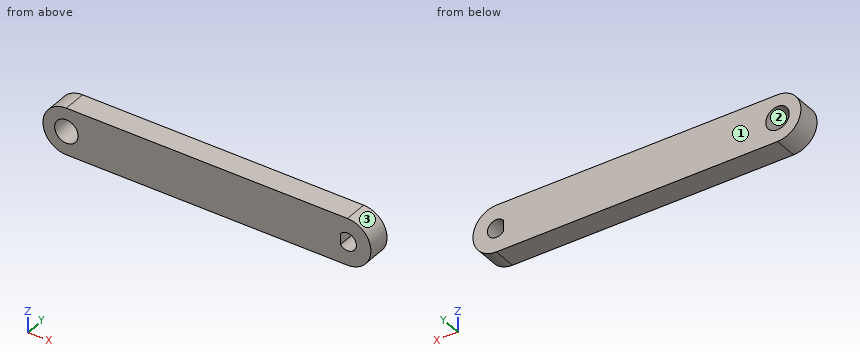
```python
from build123d import *

# Parameters (mm, degrees)
BOSS_EXTRUDE1_DEPTH = 6.35
CUT_EXTRUDE1_DEPTH  = 84.037024874
SKETCH4_R           = 3.175
CUT_EXTRUDE3_DEPTH  = 84.037024874


with BuildPart() as part:
    # Sketch1 → Boss-Extrude1 (new body)
    with BuildSketch(Plane(origin=(0, 0, 0), x_dir=(1, 0, 0), z_dir=(0, 1, 0))):
        with BuildLine():
            Line((0, -6.35), (-76.2, -6.35))
            ThreePointArc((-76.2, -6.35), (-82.55, 0), (-76.2, 6.35))
            Line((-76.2, 6.35), (0, 6.35))
            ThreePointArc((0, 6.35), (6.35, 0), (0, -6.35))
        make_face()
    extrude(amount=BOSS_EXTRUDE1_DEPTH)

    # Sketch2 → Cut-Extrude1 (cut, through all)
    with BuildSketch(Plane(origin=(0, 6.35, 0), x_dir=(1, 0, 0), z_dir=(0, 1, 0))):
        with BuildLine():
            Line((-1.905, -1.481061781), (-1.905, 1.481061781))
            ThreePointArc((-1.905, 1.481061781), (2.413, 0), (-1.905, -1.481061781))
        make_face()
    extrude(amount=-CUT_EXTRUDE1_DEPTH, mode=Mode.SUBTRACT)

    # Sketch4 → Cut-Extrude3 (cut, through all)
    with BuildSketch(Plane(origin=(0, 6.35, 0), x_dir=(1, 0, 0), z_dir=(0, 1, 0))):
        with Locations(Location((-76.2, 0, 0), (0, 0, 270))):
            Circle(SKETCH4_R)
    extrude(amount=-CUT_EXTRUDE3_DEPTH, mode=Mode.SUBTRACT)


solid = part.part
```
Build history of the part. All positions in model axes, mm. Face numbers are marked on the shaded views. Give positions to 0.01 mm unless a question says otherwise; leave off trailing zeros. Order: outer loops, then holes, each group sorted by start corner. A loop starts at its lowest first (then second) coordinate and runs counter-clockwise, first axis right, second up. Notation, with made-up numbers: M 26,-33 L 84,-33 A30 cw 84,-4 Z; hole C -38.5,36 d6. An arc over 180 degrees is marked long. Write item = value, one per line. Start each with the question number.
(1) Slice it at B-B on y = 1.5. Write the cut outline in (x, z) (3 decimals).
(2) Pin check, flat tips, straight feed: pin 1 Ø5 at (x, z) = (-76.2, 0) entering from +Y; pin 2 Ø1 at (y, z) = (3, 4) entering from +X; pin 3 Ø1.5 at (y, z) = (3.5, 2) entering from +X; pin 4 Ø1.5 at (y, z) = (2, -2.5) entering from -X. Stop position of each tip, or through.
(3) Two-plate mould, pull along X, no slides. Class the marked faces 1, 2 and 3: released by +X, released by -X, zero draft, split by the parting line, or undercut.
(4) Probe L1, parallel to X at y = 2.25, z = 0 (3 decimals); L2, parallel to X at y = 2, z = -1.25 (3 decimals); L3, parallel to X at y = 2.75, z = 2.75. List the from-to ranges inside material, lowest first. Write a range as [from, to].
(5) Slice it at A-A on z = 0. Write the cut outline in (x, y) (3 decimals).
Responses:
q1.outline = M -76.2,-6.35 L 0,-6.35 A6.35 ccw 0,6.35 L -76.2,6.35 A6.35 ccw Z; hole C -76.2,0 d6.35; hole M -1.905,-1.481 A2.413 ccw long -1.905,1.481 Z
q2.pin_1 = through
q2.pin_2 = 5.3
q2.pin_3 = 6.23
q2.pin_4 = -82.3
q3.face_1 = zero draft
q3.face_2 = undercut
q3.face_3 = released by +X
q4.L1 = [-82.55, -79.375], [-73.025, -1.905], [2.413, 6.35]
q4.L2 = [-82.426, -79.119], [-73.281, -1.905], [2.064, 6.226]
q4.L3 = [-81.92, -77.79], [-74.61, 5.72]
q5.outline = M -82.55,0 L -79.375,0 L -79.375,6.35 L -82.55,6.35 Z; M -73.025,0 L -1.905,0 L -1.905,6.35 L -73.025,6.35 Z; M 2.413,0 L 6.35,0 L 6.35,6.35 L 2.413,6.35 Z
